from build123d import *

# Parameters (mm, degrees)
SKETCH1_W           = 110
SKETCH1_H           = 125
BOSS_EXTRUDE2_DEPTH = 8
SKETCH2_R           = 2.75
CUT_EXTRUDE1_DEPTH  = 8
SKETCH3_R           = 2.5
CUT_EXTRUDE2_DEPTH  = 15
SKETCH4_R           = 2.5
CUT_EXTRUDE3_DEPTH  = 15
SKETCH5_R           = 5
CUT_EXTRUDE4_DEPTH  = 5.7


with BuildPart() as part:
    # Sketch1 → Boss-Extrude2 (new body)
    with BuildSketch(Plane(origin=(0, 0, 0), x_dir=(1, 0, 0), z_dir=(0, 1, 0))):
        Rectangle(SKETCH1_W, SKETCH1_H)
    extrude(amount=BOSS_EXTRUDE2_DEPTH)

    # Sketch2 → Cut-Extrude1 (cut)
    with BuildSketch(Plane(origin=(0, 8, 0), x_dir=(1, 0, 0), z_dir=(0, 1, 0))):
        with Locations((47, 7.5)):
            Circle(SKETCH2_R)
        with Locations((11, -7.5)):
            Circle(SKETCH2_R)
    extrude(amount=-CUT_EXTRUDE1_DEPTH, mode=Mode.SUBTRACT)

    # Sketch3 → Cut-Extrude2 (cut)
    with BuildSketch(Plane.ZY.offset(55)):
        with Locations((47.5, 4)):
            Circle(SKETCH3_R)
        with Locations((-47.5, 4)):
            Circle(SKETCH3_R)
    extrude(amount=-CUT_EXTRUDE2_DEPTH, mode=Mode.SUBTRACT)

    # Sketch4 → Cut-Extrude3 (cut)
    with BuildSketch(Plane(origin=(55, 0, 0), x_dir=(0, 0, -1), z_dir=(1, 0, 0))):
        with Locations((47.5, 4)):
            Circle(SKETCH4_R)
        with Locations((-47.5, 4)):
            Circle(SKETCH4_R)
    extrude(amount=-CUT_EXTRUDE3_DEPTH, mode=Mode.SUBTRACT)

    # Sketch5 → Cut-Extrude4 (cut)
    with BuildSketch(Plane(origin=(0, 8, 0), x_dir=(1, 0, 0), z_dir=(0, 1, 0))):
        with Locations((11, -7.5)):
            Circle(SKETCH5_R)
        with Locations((47, 7.5)):
            Circle(SKETCH5_R)
    extrude(amount=-CUT_EXTRUDE4_DEPTH, mode=Mode.SUBTRACT)


solid = part.part
Read the model definition and answer for the solid it produces. Units are mm, in the model's axes. A direction names the side the tool comes from. Round coordinates to 2 decimals unless told otherwise and drop trailing zeros. Write each loop counter-clockwise with the first axis right and the second up, starting at its lowest first coordinate (ties: lowest second). Pieces come first, ordered by that corner, then holes. Notation, with made-up numbers: (60.5, 13.25) - (85.5, 13.25) arc R27 cw to (85.5, 42.25) - close; hole circle Ø6 at (18, 65.5). An arc over 180 degrees is marked (long way). One line per question, with ' | ' between items. Start each with the question number.
1. For faces 1 (the face through (42.005, 5.19, -7.72)), 2 (the face through (47.6, 3.04, 45.19)), 3 (the face through (55, 4, 1)), 4 (the face through (-40, 4, -48)), determine the directions among +Z, -Z, +X, -X, +Y, -Y from which every point of the face is accessible in a straight line to the end or side of a thin tool.
2. Find the intervals of material crossed by probe 1 along Y at (x, z) = (-45.25, -47.5); probe 2 along X at (y, z) = (0.75, -7.5); probe 3 along Z at (x, y) = (42, 1.75), in increasing order. Write a range as [from, to].
3. Section B-B (x = 11) is taken. Determine the outline of the cut face in (y, z), and give its area (3 significant figures).
4. Section A-A (x = 47) is taken. Determine the outline of the cut face in (y, z).
5. For a pull along Y with two mould halves and no side action, classify faces 5 (the face through (15.77, 5.19, 6)), 6 (the face through (13, 2.3, 10)), 7 (the face through (-40, 4, 47)) as +Y half, -Y half, draft (parallel to the pull), parting line (faces both ways), or undercut.
6. Section D-D (z = 47.5) is taken. Determine the outline of the cut face in (x, y).
7. Section C-C (z = 7.5) is taken. Determine the outline of the cut face in (x, y), and give its area (3 significant figures).
8. Each of these flat-tipped pins is pushed along its axis until it touches: pin 1 (1.5 mm diameter, centred on y = 3.5, z = -46.5, fed in from -X); pin 2 (2.5 mm diameter, centred on y = 3.5, z = -47.5, fed in from +X); pin 3 (5 mm diameter, centred on x = 10.5, z = 8.5, fed in from +Y); pin 4 (5 mm diameter, centred on x = 47, z = -7.5, fed in from -Y). Where does it stop, or does it pass through?
Filled in:
1) face 1: +Y | face 2: +X | face 3: +Z, -Z, +X, +Y, -Y | face 4: -X
2) probe 1: [0, 1.5], [6.5, 8] | probe 2: [-55, 44.25], [49.75, 55] | probe 3: [-62.5, -48.59], [-46.41, 46.41], [48.59, 62.5]
3) outline: (0, -62.5) - (8, -62.5) - (8, 2.5) - (2.3, 2.5) - (2.3, 4.75) - (0, 4.75) - close; (0, 10.25) - (2.3, 10.25) - (2.3, 12.5) - (8, 12.5) - (8, 62.5) - (0, 62.5) - close | area: 930 mm²
4) outline: (0, -62.5) - (8, -62.5) - (8, -12.5) - (2.3, -12.5) - (2.3, -10.25) - (0, -10.25) - close; (0, -4.75) - (2.3, -4.75) - (2.3, -2.5) - (8, -2.5) - (8, 62.5) - (0, 62.5) - close; hole circle Ø5 at (4, -47.5); hole circle Ø5 at (4, 47.5)
5) face 5: draft | face 6: +Y half | face 7: undercut
6) outline: (-55, 0) - (55, 0) - (55, 1.5) - (40, 1.5) - (40, 6.5) - (55, 6.5) - (55, 8) - (-55, 8) - (-55, 6.5) - (-40, 6.5) - (-40, 1.5) - (-55, 1.5) - close
7) outline: (-55, 0) - (8.25, 0) - (8.25, 2.3) - (6, 2.3) - (6, 8) - (-55, 8) - close; (13.75, 0) - (55, 0) - (55, 8) - (16, 8) - (16, 2.3) - (13.75, 2.3) - close | area: 810 mm²
8) pin 1: x = -40 | pin 2: x = 40 | pin 3: y = 2.3 | pin 4: through
